Verification items for the finished model (mm, model axes). A direction names the side the tool comes from. Round coordinates to 2 decimals unless told otherwise and drop trailing zeros. Order: outer loops, then holes, each group sorted by start corner. A loop starts at its lowest first (then second) coordinate and runs counter-clockwise, first axis right, second up. Notation, with made-up numbers: (19, -28.75) -> (58, -28.75) arc R23 cw to (58, -16.75) -> close; hole circle Ø10 at (15, 73). An arc over 180 degrees is marked (long way). Return JSON: item names as keys, results as strings. Group by question number.
Item 1: Scan lines: probe 1 along X at (y, z) = (-10.05, -14.5); probe 2 along Z at (x, y) = (0.5, 9.5); probe 3 along Y at (x, z) = (-16.5, -1.5). Record each from-to range of solid material in increasing order. Write a range as from..to.
Item 2: Sectioned sample at A-A on z = -33. Record the cut outline in (x, y).
Item 3: Sectioned sample at C-C on x = -18.5. Record the cut outline in (y, z).
Item 4: Sectioned sample at B-B on x = 0. Record the cut outline in (y, z).
Item 5: Draft check along X on faces 6 (the cylindrical face through (0, -0.9, 34.2)), 7 (the flat face through (-1, 0, 30)), 8 (the cylindrical face through (17.657, -9.726, 16.532)). Enter one of: pulls with the +X half, pulls with the -X half, needs draft (parallel to the pull), parting line crosses it, or undercut.
Item 6: Access from +Z, -Z, +X, -X, +Y, -Y to the whole of each face (thin tool, end or side, straight path). Record for faces 1 (the flat face through (-1, 0, -30)), 2 (the flat face through (1, 0, 30)), 3 (the flat face through (1, 0, -30)), 4 (the flat face through (0, 1, -27)), 5 (the flat face through (0, -1, 27)).
Item 7: Depth check by flat-ended pin: pin 1 Ø2.5 at (x, z) = (-18.5, -14.5) entering from -Y; pin 2 Ø1.6 at (x, z) = (0, -32.5) entering from +Y; pin 3 Ø2 at (x, y) = (-7, 7.5) entering from -Z; pin 4 Ø1.6 at (x, z) = (0, -26.5) entering from +Y. Enter the tip coordinate at first touch or a pass-through.
Item 8: Sectioned sample at D-D on z = -14.5. Record the cut outline in (x, y).
```python
from build123d import *

# Parameters (mm, degrees)
BOSS_EXTRUDE1_DEPTH = 24.5
SKETCH2_R           = 2.2
CUT_EXTRUDE1_DEPTH  = 40.956226048
SKETCH3_R           = 1.5
BOSS_EXTRUDE2_DEPTH = 1


with BuildPart() as part:
    # Sketch1 → Boss-Extrude1 (new, symmetric)
    with BuildSketch(Plane.XY):
        with BuildLine():
            Line((12.5, -8), (24, -8))
            Line((24, -8), (24, -11.5))
            Line((24, -11.5), (-24, -11.5))
            Line((-24, -11.5), (-24, -8))
            Line((-24, -8), (-12.5, -8))
            Line((-12.5, -8), (-12.5, 0))
            ThreePointArc((-12.5, 0), (0, 12.5), (12.5, 0))
            Line((12.5, 0), (12.5, -8))
        make_face()
    extrude(amount=BOSS_EXTRUDE1_DEPTH, both=True)

    # Sketch2 → Cut-Extrude1 (cut, through all)
    with BuildSketch(Plane(origin=(0, -8, 0), x_dir=(1, 0, 0), z_dir=(0, 1, 0))):
        with Locations(Location((-18.5, 14.5, 0), (0, 0, 270))):
            Circle(SKETCH2_R)
        with Locations(Location((-18.5, -14.5, 0), (0, 0, 270))):
            Circle(SKETCH2_R)
        with Locations(Location((18.5, -14.5, 0), (0, 0, 270))):
            Circle(SKETCH2_R)
        with Locations(Location((18.5, 14.5, 0), (0, 0, 270))):
            Circle(SKETCH2_R)
    extrude(amount=-CUT_EXTRUDE1_DEPTH, mode=Mode.SUBTRACT)

    # Sketch3 → Boss-Extrude2 (add, symmetric)
    # profile 1 of 2: a face of its own
    with BuildSketch(Plane(origin=(0, 0, 0), x_dir=(0, 0, -1), z_dir=(1, 0, 0))):
        Polygon((-29.5, -1), (-24.5, -1), (-24.5, 1), (-29.5, 1), (-30.5, 2), (-35.5, 2), (-35.5, -2), (-30.5, -2), align=None)
        with Locations((-33, 0)):
            Circle(SKETCH3_R, mode=Mode.SUBTRACT)
    # profile 2 of 2: a face of its own
    with BuildSketch(Plane(origin=(0, 0, 0), x_dir=(0, 0, -1), z_dir=(1, 0, 0))):
        Polygon((24.5, -1), (24.5, 1), (29.5, 1), (30.5, 2), (35.5, 2), (35.5, -2), (30.5, -2), (29.5, -1), align=None)
        with Locations((33, 0)):
            Circle(SKETCH3_R, mode=Mode.SUBTRACT)
    extrude(amount=BOSS_EXTRUDE2_DEPTH, both=True)


solid = part.part
```
Recorded:
{
 "1": {"probe 1": "-24..-20.7, -16.3..16.3, 20.7..24", "probe 2": "-24.5..24.5", "probe 3": "-11.5..-8"},
 "2": {"outline": "(-1, -2) -> (1, -2) -> (1, -1.5) -> (-1, -1.5) -> close; (-1, 1.5) -> (1, 1.5) -> (1, 2) -> (-1, 2) -> close"},
 "3": {"outline": "(-11.5, -24.5) -> (-8, -24.5) -> (-8, -16.7) -> (-11.5, -16.7) -> close; (-11.5, -12.3) -> (-8, -12.3) -> (-8, 12.3) -> (-11.5, 12.3) -> close; (-11.5, 16.7) -> (-8, 16.7) -> (-8, 24.5) -> (-11.5, 24.5) -> close"},
 "4": {"outline": "(-11.5, -24.5) -> (-1, -24.5) -> (-1, -29.5) -> (-2, -30.5) -> (-2, -35.5) -> (2, -35.5) -> (2, -30.5) -> (1, -29.5) -> (1, -24.5) -> (12.5, -24.5) -> (12.5, 24.5) -> (1, 24.5) -> (1, 29.5) -> (2, 30.5) -> (2, 35.5) -> (-2, 35.5) -> (-2, 30.5) -> (-1, 29.5) -> (-1, 24.5) -> (-11.5, 24.5) -> close; hole circle Ø3 at (0, -33); hole circle Ø3 at (0, 33)"},
 "5": {"face 6": "needs draft", "face 7": "pulls with the -X half", "face 8": "undercut"},
 "6": {"face 1": "-Z, -X, +Y, -Y", "face 2": "+Z, +X, +Y, -Y", "face 3": "-Z, +X, +Y, -Y", "face 4": "+X, -X, +Y", "face 5": "+X, -X, -Y"},
 "7": {"pin 1": "through", "pin 2": "y = 2", "pin 3": "z = -24.5", "pin 4": "y = 1"},
 "8": {"outline": "(-24, -11.5) -> (-20.7, -11.5) -> (-20.7, -8) -> (-24, -8) -> close; (-16.3, -11.5) -> (16.3, -11.5) -> (16.3, -8) -> (12.5, -8) -> (12.5, 0) arc R12.5 ccw to (-12.5, 0) -> (-12.5, -8) -> (-16.3, -8) -> close; (20.7, -11.5) -> (24, -11.5) -> (24, -8) -> (20.7, -8) -> close"}
}
